Check sheet for the modelled part. Datum: model origin and axes. Units: mm. A direction names the side the tool comes from. Give positions to 0.01 mm unless a question says otherwise; leave off trailing zeros. Order: outer loops, then holes, each group sorted by start corner. A loop starts at its lowest first (then second) coordinate and runs counter-clockwise, first axis right, second up. Notation, with made-up numbers: (23.5, -15.75) -> (65.5, -15.75) arc R11 cw to (65.5, -2.75) -> close; hole circle Ø1 at (-32, 71.5). An arc over 180 degrees is marked (long way). Write each question's results on one line, items separated by ' | '.
from build123d import *

# Parameters (mm, degrees)
SKETCH_1_W          = 34
SKETCH_1_H          = 38
SKETCH_1_W_2        = 28
SKETCH_1_H_2        = 28
SKETCH_1_H_3        = 15
SKETCH_1_R          = 1.5
EXTRUDE_1_DEPTH     = 3
SKETCH_2_R          = 2.5
EXTRUDE_2_DEPTH     = 12
SKETCH_3_R          = 1
CUT_EXTRUDE_1_DEPTH = 8
FILLET_1_R          = 4
SKETCH_4_W          = 12
SKETCH_4_H          = 5
CUT_EXTRUDE_2_DEPTH = 8


with BuildPart() as part:
    # 草图1 → 凸台-拉伸1 (new body)
    # profile 1 of 3: a face of its own
    with BuildSketch(Plane.XY):
        with Locations((0, 26.5)):
            Rectangle(SKETCH_1_W, SKETCH_1_H)
        with Locations((0, 28.5)):
            Rectangle(SKETCH_1_W_2, SKETCH_1_H_2, mode=Mode.SUBTRACT)
    # profile 2 of 3: a face of its own
    with BuildSketch(Plane.XY):
        with Locations((0, 28.5)):
            Rectangle(SKETCH_1_W_2, SKETCH_1_H_2)
    # profile 3 of 3: a face of its own
    with BuildSketch(Plane.XY):
        Rectangle(SKETCH_1_W, SKETCH_1_H_3)
        with Locations((13.5, 0)):
            Circle(SKETCH_1_R, mode=Mode.SUBTRACT)
        with Locations((-13.5, 0)):
            Circle(SKETCH_1_R, mode=Mode.SUBTRACT)
    extrude(amount=EXTRUDE_1_DEPTH)

    # 草图2 → 凸台-拉伸2 (add)
    with BuildSketch(Plane.XY.offset(3)):
        with Locations((-14, 42.5)):
            Circle(SKETCH_2_R)
        with Locations((14, 42.5)):
            Circle(SKETCH_2_R)
        with Locations((-14, 14.5)):
            Circle(SKETCH_2_R)
        with Locations((14, 14.5)):
            Circle(SKETCH_2_R)
    extrude(amount=EXTRUDE_2_DEPTH)

    # 草图3 → 切除-拉伸1 (cut)
    with BuildSketch(Plane.XY.offset(15)):
        with Locations((-14, 42.5)):
            Circle(SKETCH_3_R)
        with Locations((14, 42.5)):
            Circle(SKETCH_3_R)
        with Locations((-14, 14.5)):
            Circle(SKETCH_3_R)
        with Locations((14, 14.5)):
            Circle(SKETCH_3_R)
    extrude(amount=-CUT_EXTRUDE_1_DEPTH, mode=Mode.SUBTRACT)

    # 圆角1
    fillet_1_edges = [part.edges().sort_by_distance(p)[0] for p in [
        (-17, 45.5, 1.5),
        (17, 45.5, 1.5),
        (17, -7.5, 1.5),
        (-17, -7.5, 1.5),
    ]]
    fillet(fillet_1_edges, radius=FILLET_1_R)

    # 草图4 → 切除-拉伸2 (cut)
    with BuildSketch(Plane.XY.offset(3)):
        with Locations((0.114195125, 18)):
            Rectangle(SKETCH_4_W, SKETCH_4_H)
    extrude(amount=-CUT_EXTRUDE_2_DEPTH, mode=Mode.SUBTRACT)


solid = part.part
1. Section check C-C on y = 0. Record the cut outline in (x, z), then the cut area to 3 significant figures.
Verdict:
outline: (-17, 0) -> (-15, 0) -> (-15, 3) -> (-17, 3) -> close; (-12, 0) -> (12, 0) -> (12, 3) -> (-12, 3) -> close; (15, 0) -> (17, 0) -> (17, 3) -> (15, 3) -> close | area: 84.0 mm^2
2. Access from +Z, -Z, +X, -X, +Y, -Y to the whole of each face (thin tool, end or side, straight path). Record for faces 1 (the flat face through (0, 20.5, 2)), 2 (the flat face through (14, 43, 7)), 3 (the flat face through (14, 13, 15)).
Verdict:
face 1: +Z, -Z | face 2: +Z | face 3: +Z, +X, -X, +Y, -Y
3. Section check A-A on z = 8.5. Record the cut outline in (x, y), then the cut area to 3 significant figures.
Verdict:
outline: circle Ø5 at (-14, 14.5); circle Ø5 at (-14, 42.5); circle Ø5 at (14, 14.5); circle Ø5 at (14, 42.5); hole circle Ø2 at (-14, 14.5); hole circle Ø2 at (-14, 42.5); hole circle Ø2 at (14, 14.5); hole circle Ø2 at (14, 42.5) | area: 66.0 mm^2
4. Gauge pin test, flat ends, axial feed: pin 1 Ø1.6 at (x, y) = (13.5, 42.5) entering from +Z; pin 2 Ø0.6 at (x, y) = (-14, 42.5) entering from +Z; pin 3 Ø6 at (y, z) = (19.5, 7.5) entering from +X; pin 4 Ø3.5 at (x, y) = (13.5, 0) entering from +Z. Record the tip position at first contact, or that the pin passes through.
Verdict:
pin 1: stops at z = 15 | pin 2: stops at z = 7 | pin 3: stops at x = 15.5 | pin 4: stops at z = 3
5. Material ranges on probe 1 along Y at (x, z) = (14, 9); probe 2 along X at (y, z) = (15, 8.75); probe 3 along Y at (x, z) = (4, 2), recorded low to high. Write a range as from..to.
Verdict:
probe 1: y = 12..13.5, 15.5..17, 40..41.5, 43.5..45 | probe 2: x = -16.45..-14.87, -13.13..-11.55, 11.55..13.13, 14.87..16.45 | probe 3: y = -7.5..15.5, 20.5..45.5
6. Section check B-B on x = 0.5. Record the cut outline in (y, z), then the cut area to 3 significant figures.
Verdict:
outline: (-7.5, 0) -> (15.5, 0) -> (15.5, 3) -> (-7.5, 3) -> close; (20.5, 0) -> (45.5, 0) -> (45.5, 3) -> (20.5, 3) -> close | area: 144 mm^2
7. Mould release check, pull along Y, two halves, no side actions. Record for faces 4 (the flat face through (0, 25, 0)), 5 (the cylindrical face through (-14.54, 40.06, 8.92)), 6 (the cylindrical face through (15.797, -6.359, 1.521)): +Y half, -Y half, draft (parallel to the pull), parting line (faces both ways), or undercut.
Verdict:
face 4: draft | face 5: undercut | face 6: -Y half
8. Section check D-D on y = 18. Record the cut outline in (x, z).
Verdict:
outline: (-17, 0) -> (-5.89, 0) -> (-5.89, 3) -> (-17, 3) -> close; (6.11, 0) -> (17, 0) -> (17, 3) -> (6.11, 3) -> close
